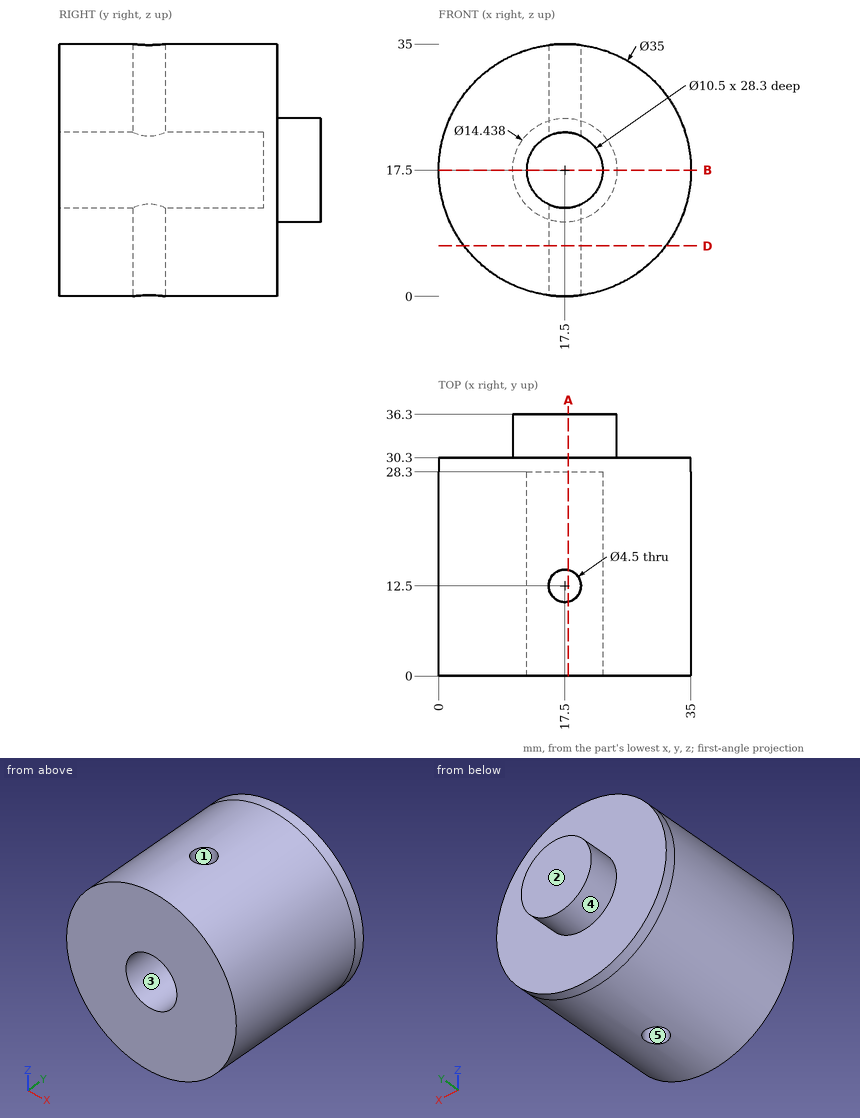
Print and shaded views of the part. All mm, measured from the part's lowest x, y and z. A direction names the side the tool comes from. Round coordinates to 2 decimals unless told otherwise and drop trailing zeros. Loops run counter-clockwise (first coordinate to the right, second up) from the corner with the lowest first, then second, coordinate; pieces in that order, holes last. Notation, with made-up numbers: M -4.5,33 L 3.5,33 A21 ccw 3.5,70 Z; hole C 88,5 d7. An arc over 180 degrees is marked long. One line per question, with ' | ' between items.
1) Flat gauge pins, fed straight in: pin 1 (6.5 mm diameter, centred on x = 17.5, z = 17.5, fed in from -Y); pin 2 (2 mm diameter, centred on x = 11.5, z = 27, fed in from +Y); pin 3 (4 mm diameter, centred on y = 16, z = 5.5, fed in from +X). Where does each tip first touch, or does it go through?
Solved:
pin 1: stops at y = 28.3 | pin 2: stops at y = 30.3 | pin 3: stops at x = 31.86
2) Band-saw the part on B-B (z = 17.5). Give the cut face in (x, y).
Solved:
outline: M 0,0 L 12.25,0 L 12.25,28.3 L 22.75,28.3 L 22.75,0 L 35,0 L 35,30.3 L 24.72,30.3 L 24.72,36.3 L 10.28,36.3 L 10.28,30.3 L 0,30.3 Z
3) Band-saw the part on D-D (z = 7). Give the cut face in (x, y).
Solved:
outline: M 3.5,0 L 31.5,0 L 31.5,30.3 L 3.5,30.3 Z; hole C 17.5,12.5 d4.5
4) Mould opens along Y. For the marked faces 1, 2 and 3 say: +Y half, -Y half, draft (parallel to the pull), parting line (faces both ways), or undercut.
Solved:
face 1: undercut | face 2: +Y half | face 3: draft
5) 3-axis set-ups, long thin cutter, end or side, ignore diameter. For the marked faces 4 and 5: which of +Z, -Z, +X, -X, +Y, -Y reach the whole face in a straight line?
Solved:
face 4: +Y | face 5: +Z, -Z
6) Band-saw the part on A-A (x = 18). Give the cut face in (y, z), then the cut area to 3 significant figures.
Solved:
outline: M 0,0.01 L 10.31,0.01 L 10.31,12.27 L 0,12.27 Z; M 0,22.73 L 10.31,22.73 L 10.31,34.99 L 0,34.99 Z; M 14.69,0.01 L 30.3,0.01 L 30.3,10.3 L 36.3,10.3 L 36.3,24.7 L 30.3,24.7 L 30.3,34.99 L 14.69,34.99 L 14.69,22.73 L 28.3,22.73 L 28.3,12.27 L 14.69,12.27 Z | area: 743 mm²
7) Drill centre lines: line 1 along Z through (x, y) = (17.5, 8.5); line 2 along Y through (x, z) = (20, 18); line 3 along Y through (x, z) = (17, 30). Where is each one in solid material? Low to high.
Solved:
line 1: z = 0 to 12.25, 22.75 to 35 | line 2: y = 28.3 to 36.3 | line 3: y = 0 to 10.31, 14.69 to 30.3
